from build123d import *

# Parameters (mm, degrees)
F0_R     = 1.5875
F0_R_2   = 38.1
F1_DEPTH = 1.5875
F3_DEPTH = 2.38125
F4_R     = 3.175
F5_DEPTH = 0.79375


with BuildPart() as f1:
    # F0 (on Top) → F1 (new body)
    with BuildSketch(Plane.XY):
        with BuildLine():
            ThreePointArc((80.7339, -39.9161), (120.65, 0), (80.7339, 39.9161))
            Line((80.7339, 39.9161), (-80.7339, 39.9161))
            ThreePointArc((-80.7339, 39.9161), (-120.65, 0), (-80.7339, -39.9161))
            Line((-80.7339, -39.9161), (80.7339, -39.9161))
        make_face()
        with Locations((-35.1536, -35.1536)):
            Circle(F0_R, mode=Mode.SUBTRACT)
        with Locations((35.1536, -35.1536)):
            Circle(F0_R, mode=Mode.SUBTRACT)
        with Locations((-35.1536, 35.1536)):
            Circle(F0_R, mode=Mode.SUBTRACT)
        Circle(F0_R_2, mode=Mode.SUBTRACT)
        with Locations((35.1536, 35.1536)):
            Circle(F0_R, mode=Mode.SUBTRACT)
    extrude(amount=F1_DEPTH)

    # F2 (on face) → F3 (join)
    with BuildSketch(Plane.XY.offset(1.5875)):
        with BuildLine():
            Line((80.7339, 39.9161), (-80.7339, 39.9161))
            ThreePointArc((-80.7339, 39.9161), (-120.65, 0), (-80.7339, -39.9161))
            Line((-80.7339, -39.9161), (80.7339, -39.9161))
            ThreePointArc((80.7339, -39.9161), (120.65, 0), (80.7339, 39.9161))
        make_face()
        with BuildLine():
            ThreePointArc((80.7339, 38.3286), (119.0625, 0), (80.7339, -38.3286))
            Line((80.7339, -38.3286), (-80.7339, -38.3286))
            ThreePointArc((-80.7339, -38.3286), (-119.0625, 0), (-80.7339, 38.3286))
            Line((-80.7339, 38.3286), (80.7339, 38.3286))
        make_face(mode=Mode.SUBTRACT)
    extrude(amount=F3_DEPTH)

    # F4 (on face) → F5 (cut)
    with BuildSketch(Plane.XY.offset(1.5875)):
        with Locations((-35.1536, 35.1536)):
            Circle(F4_R)
        with Locations((35.1536, 35.1536)):
            Circle(F4_R)
        with Locations((35.1536, -35.1536)):
            Circle(F4_R)
        with Locations((-35.1536, -35.1536)):
            Circle(F4_R)
    extrude(amount=-F5_DEPTH, mode=Mode.SUBTRACT)


solid = f1.part
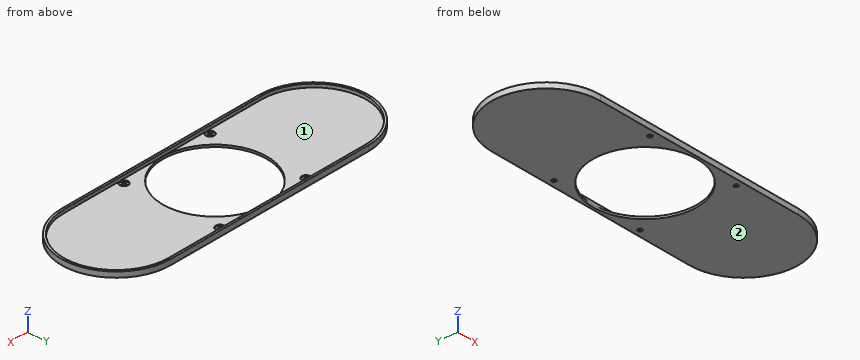
Input: part model. Units: mm. Frame: model coordinates. Face numbers are marked on the shaded views. Coordinates: 2 decimals unless noted, no trailing zeros. Loops run counter-clockwise (first coordinate to the right, second up) from the corner with the lowest first, then second, coordinate; pieces in that order, holes last. Notation, with made-up numbers: (57.5, 51) -> (82.5, 51) arc R12 ccw to (82.5, 55) -> close; hole circle Ø6 at (2, 30). An arc over 180 degrees is marked (long way). Write item = value, one per line. Start each with the question number.
Item 1: Cut plane B-B, the plane y = 0. Return loops of the section in (x, z), plus the area to 3 significant figures.
Item 2: Cut plane D-D, the plane x = 94.5. Return loops of the section in (y, z), plus the area to 3 significant figures.
Item 3: Material intervals for line 1 (Y direction, x = 69, z = 3.3); line 2 (X direction, y = 33, z = 1.05); line 3 (Z direction, x = -81.5, y = 13), sorted ascending.
Item 4: Mould query, pull axis Y, two halves, no side actions, for the marked faces 1 and 2. Classes: pulls with the +Y half, pulls with the -Y half, needs draft (parallel to the pull), parting line crosses it, or undercut.
Item 5: Cut plane A-A, the plane x = 0. Return loops of the section in (y, z).
Item 6: Cut plane C-C, the plane z = 3. Return loops of the section in (x, y), plus the area to 3 significant figures.
Item 7: First-contact query: P1, Ø12, axis at x = -56.5, y = 31, coming from the -Z side; P2, Ø5, axis at x = 35.5, y = -34, coming from the +Z side; P3, Ø3.5, axis at x = -35.15, y = -35.15, coming from the +Z side. Flat tips, straight axial feed; report the tip coordinate or a pass-through.
Ans:
q1.outline = (-120.65, 0) -> (-38.1, 0) -> (-38.1, 1.59) -> (-119.06, 1.59) -> (-119.06, 3.97) -> (-120.65, 3.97) -> close; (38.1, 0) -> (120.65, 0) -> (120.65, 3.97) -> (119.06, 3.97) -> (119.06, 1.59) -> (38.1, 1.59) -> close
q1.area = 270 mm²
q2.outline = (-37.47, 0) -> (37.47, 0) -> (37.47, 3.97) -> (35.77, 3.97) -> (35.77, 1.59) -> (-35.77, 1.59) -> (-35.77, 3.97) -> (-37.47, 3.97) -> close
q2.area = 127 mm²
q3.line_1 = -39.92 to -38.33, 38.33 to 39.92
q3.line_2 = -103.19 to -37.49, -32.82 to -19.04, 19.04 to 32.82, 37.49 to 103.19
q3.line_3 = 0 to 1.59
q4.face_1 = undercut
q4.face_2 = needs draft
q5.outline = (-39.92, 0) -> (-38.1, 0) -> (-38.1, 1.59) -> (-38.33, 1.59) -> (-38.33, 3.97) -> (-39.92, 3.97) -> close; (38.1, 0) -> (39.92, 0) -> (39.92, 3.97) -> (38.33, 3.97) -> (38.33, 1.59) -> (38.1, 1.59) -> close
q6.outline = (-80.73, -39.92) -> (80.73, -39.92) arc R39.92 ccw to (80.73, 39.92) -> (-80.73, 39.92) arc R39.92 ccw to start; hole (-80.73, -38.33) -> (80.73, -38.33) arc R38.33 ccw to (80.73, 38.33) -> (-80.73, 38.33) arc R38.33 ccw to start
q6.area = 903 mm²
q7.P1 = 0
q7.P2 = 1.59
q7.P3 = 0.79
